from build123d import *

# Parameters (mm, degrees)
SKETCH1_R               = 9.5
SKETCH1_R_2             = 6.35
BOSS_EXTRUDE1_DEPTH     = 27.5
CUT_EXTRUDE2_DEPTH      = 91.767085063
CUT_EXTRUDE2_DEPTH_BACK = 6
CUT_EXTRUDE3_DEPTH      = 91.767085063
CUT_EXTRUDE3_DEPTH_BACK = 6
CUT_EXTRUDE5_DEPTH      = 6.75
CUT_EXTRUDE5_DEPTH_BACK = 6.75


with BuildPart() as part:
    # Sketch1 → Boss-Extrude1 (new body)
    with BuildSketch(Plane(origin=(0, 0, 0), x_dir=(0, 0, -1), z_dir=(1, 0, 0))):
        with BuildLine():
            Line((39, 6.5), (61, 6.5))
            Line((61, 6.5), (61, 15))
            ThreePointArc((61, 15), (24.894386745, 25.257382556), (-0.029226303, 53.322355709))
            ThreePointArc((-0.029226303, 53.322355709), (-16.577537576, 60.777514808), (-26.578667772, 45.631446077))
            Line((-26.578667772, 45.631446077), (-21, 0))
            ThreePointArc((-21, 0), (-14.849242405, -14.849242405), (0, -21))
            Line((0, -21), (61, -21))
            Line((61, -21), (61, -6.5))
            Line((61, -6.5), (39, -6.5))
            ThreePointArc((39, -6.5), (32.5, 0), (39, 6.5))
        make_face()
        Circle(SKETCH1_R, mode=Mode.SUBTRACT)
        with Locations((-12.68213321, 47.330365488)):
            Circle(SKETCH1_R_2, mode=Mode.SUBTRACT)
    extrude(amount=BOSS_EXTRUDE1_DEPTH)

    # Sketch4 → Cut-Extrude2 (cut, two sides: drawn at the far end of the back side and taken through both)
    with BuildSketch(Plane.ZY.offset(-CUT_EXTRUDE2_DEPTH_BACK)):
        with BuildLine():
            Line((-222.712922977, 38.330365488), (-9.709497533, 38.330365488))
            Line((-9.709497533, 38.330365488), (-4.051067321, 38.330365488))
            ThreePointArc((-4.051067321, 38.330365488), (9.181632836, 28.655609877), (25.019880988, 32.881144756))
            Line((25.019880988, 32.881144756), (187.005855245, 171.196015234))
            Line((187.005855245, 171.196015234), (55.595163053, 576.428130178))
            Line((55.595163053, 576.428130178), (-354.123615169, 443.562480432))
            Line((-354.123615169, 443.562480432), (-222.712922977, 38.330365488))
        make_face()
    extrude(amount=CUT_EXTRUDE2_DEPTH + CUT_EXTRUDE2_DEPTH_BACK, mode=Mode.SUBTRACT)

    # Sketch6 → Cut-Extrude3 (cut, two sides: drawn at the far end of the back side and taken through both)
    with BuildSketch(Plane(origin=(27.5, 0, 0), x_dir=(0, 0, -1), z_dir=(1, 0, 0)).offset(-CUT_EXTRUDE3_DEPTH_BACK)):
        with BuildLine():
            Line((-187.005855245, 171.196015234), (-25.019880988, 32.881144756))
            ThreePointArc((-25.019880988, 32.881144756), (-9.181632836, 28.655609877), (4.051067321, 38.330365488))
            Line((4.051067321, 38.330365488), (9.709497533, 38.330365488))
            Line((9.709497533, 38.330365488), (222.712922977, 38.330365488))
            Line((222.712922977, 38.330365488), (354.123615169, 443.562480432))
            Line((354.123615169, 443.562480432), (-55.595163053, 576.428130178))
            Line((-55.595163053, 576.428130178), (-187.005855245, 171.196015234))
        make_face()
    extrude(amount=CUT_EXTRUDE3_DEPTH + CUT_EXTRUDE3_DEPTH_BACK, mode=Mode.SUBTRACT)

    # Sketch12 → Cut-Extrude5 (cut, two sides: drawn at the far end of the back side and taken through both)
    with BuildSketch(Plane(origin=(13.75, 0, 0), x_dir=(0, 0, -1), z_dir=(1, 0, 0)).offset(-CUT_EXTRUDE5_DEPTH_BACK)):
        with BuildLine():
            ThreePointArc((61, 15), (41.129282246, 17.866834211), (23, 26.491988568))
            Line((23, 26.491988568), (23, -21))
            Line((23, -21), (61, -21))
            Line((61, -21), (61, -6.5))
            Line((61, -6.5), (39, -6.5))
            ThreePointArc((39, -6.5), (32.5, 0), (39, 6.5))
            Line((39, 6.5), (61, 6.5))
            Line((61, 6.5), (61, 15))
        make_face()
    extrude(amount=CUT_EXTRUDE5_DEPTH + CUT_EXTRUDE5_DEPTH_BACK, mode=Mode.SUBTRACT)


solid = part.part
Source: CAD feature listing. Evaluate the final solid. Frame: model axes, mm. A direction names the side the tool comes from. Coordinates: 2 decimals unless noted, no trailing zeros. Loops run counter-clockwise (first coordinate to the right, second up) from the corner with the lowest first, then second, coordinate; pieces in that order, holes last. Notation, with made-up numbers: (-17.5, 55.5) - (23.5, 55.5) arc R19 ccw to (23.5, 91.5) - close; hole circle Ø3 at (50.5, 52). An arc over 180 degrees is marked (long way). One line per item, written item: value. Start each with the question number.
1. Section D-D (z = -51). Return the cut outline in (x, y).
2. Ray query, L1, parallel to X at y = 9.5, z = -49; L2, parallel to X at y = 42.5, z = 2; L3, parallel to Y at x = 15, z = 6. Return the intervals inside material, ascending.
3. Section B-B (x = 2). Return the cut outline in (y, z).
4. Section A-A (y = -2.5). Return the cut outline in (x, z).
5. Mould query, pull axis Y, two halves, no side actions, for faces 1 (the flat face through (0, 2, -17)), 2 (the cylindrical face through (13.558, -14.685, 15.012)), 3 (the cylindrical face through (13.642, 51.622, 17.362)). Classes: pulls with the +Y half, pulls with the -Y half, needs draft (parallel to the pull), parting line crosses it, or undercut.
6. Section C-C (z = 8.5). Return the cut outline in (x, y), and give its area (3 significant figures).
7. Contact query for flat-ended pins moving along their axis: P1, Ø7.5, axis at x = 3, z = -51, coming from the +Y side; P2, Ø3, axis at x = 3.5, z = -5.5, coming from the +Y side; P3, Ø3, axis at x = 12, z = -7, coming from the +Y side; P4, Ø3, axis at y = 44, z = 14.5, coming from the +X side. Output: stop coordinate, or through.
8. Set-up query: faces 4 (the cylindrical face through (3.04, 28.7, 8.95)), 5 (the flat face through (24, 6.5, -50)), 6 (the cylindrical face through (24.458, 28.613, 9.415)), 7 (the flat face through (14, 3, -23)), 8 (the flat face through (13.558, 18.065, 23.209)). Return all of +Z, -Z, +X, -X, +Y, -Y with unobstructed straight access to the full face (end or side cutting, diameter ignored); none if empty.
Verdict:
1. outline: (0, -21) - (7, -21) - (7, -6.5) - (0, -6.5) - close; (0, 6.5) - (7, 6.5) - (7, 15.68) - (0, 15.68) - close; (20.5, -21) - (27.5, -21) - (27.5, -6.5) - (20.5, -6.5) - close; (20.5, 6.5) - (27.5, 6.5) - (27.5, 15.68) - (20.5, 15.68) - close
2. L1: x = 0 to 7, 20.5 to 27.5
2. L2: x = 6 to 21.5
2. L3: y = -20.12 to -7.37, 7.37 to 59.63
3. outline: (-21, -61) - (-6.5, -61) - (-6.5, -39) arc R6.5 cw to (6.5, -39) - (6.5, -61) - (15, -61) arc R67 cw to (38.33, -9.71) - (38.33, -4.05) arc R19 cw to (32.88, 25.02) - (0, 21) arc R21 ccw to (-21, 0) - close; hole circle Ø19 at (0, 0)
4. outline: (0, -33) - (7, -33) - (7, -23) - (20.5, -23) - (20.5, -33) - (27.5, -33) - (27.5, -9.17) - (0, -9.17) - close; (0, 9.17) - (27.5, 9.17) - (27.5, 20.85) - (0, 20.85) - close
5. face 1: needs draft
5. face 2: pulls with the -Y half
5. face 3: undercut
6. outline: (0, -19.2) - (27.5, -19.2) - (27.5, -4.24) - (0, -4.24) - close; (0, 4.24) - (27.5, 4.24) - (27.5, 28.8) - (21.5, 28.8) - (21.5, 42.55) - (6, 42.55) - (6, 28.8) - (0, 28.8) - close; (6, 52.11) - (21.5, 52.11) - (21.5, 60.69) - (6, 60.69) - close
6. area: 1,430 mm2
7. P1: stops at y = 16.33
7. P2: stops at y = 38.33
7. P3: stops at y = 43.77
7. P4: passes through
8. face 4: -X, +Y
8. face 5: -Z, +X, -X
8. face 6: +X, +Y
8. face 7: -Z, +Y, -Y
8. face 8: +Z, +X, -X, -Y
